Verification items for the finished model (mm, model axes). Face numbers are marked on the shaded views. A direction names the side the tool comes from. Round coordinates to 2 decimals unless told otherwise and drop trailing zeros. Write each loop counter-clockwise with the first axis right and the second up, starting at its lowest first coordinate (ties: lowest second). Pieces come first, ordered by that corner, then holes. Notation, with made-up numbers: (64.25, 75) - (113.25, 75) arc R6 ccw to (113.25, 79) - close; hole circle Ø7 at (38, 85). An arc over 180 degrees is marked (long way). Write each question's results on one line, items separated by ' | '.
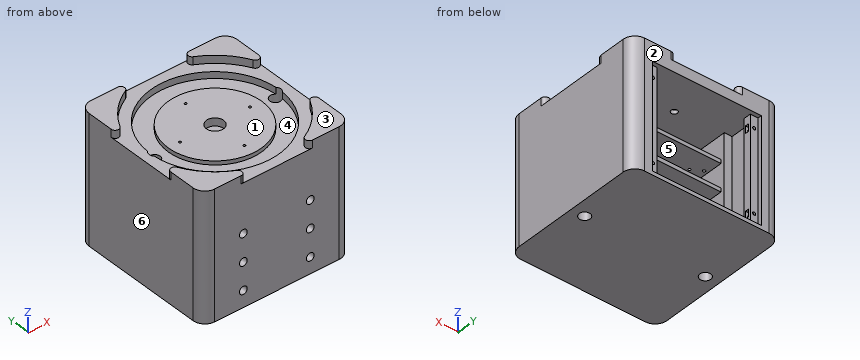
```python
from build123d import *

# Parameters (mm, degrees)
SKETCH_W             = 190
SKETCH_H             = 190
PAD_DEPTH            = 165
SKETCH001_R          = 82.5
POCKET_DEPTH         = 20
SKETCH002_R          = 60
PAD001_DEPTH         = 5
FILLET_R             = 15
SKETCH003_W          = 100
SKETCH003_H          = 30
POCKET001_DEPTH      = 160
SKETCH004_W          = 120
SKETCH004_H          = 135
POCKET002_DEPTH      = 50
SKETCH005_R          = 1.5
POCKET003_DEPTH      = 10
SKETCH006_R          = 4
POCKET004_DEPTH      = 5
SKETCH007_R          = 11
POCKET005_DEPTH      = 10
SKETCH008_W          = 140
SKETCH008_H          = 135
POCKET006_DEPTH      = 5
SKETCH009_W          = 30
SKETCH009_H          = 135
POCKET007_DEPTH      = 10
SKETCH010_W          = 30
SKETCH010_H          = 135
POCKET008_DEPTH      = 10
SKETCH011_W          = 304.305817
SKETCH011_H          = 239.475426
POCKET009_DEPTH      = 1.5
SKETCH012_R          = 96
SKETCH012_R_2        = 75
POCKET010_DEPTH      = 10
FILLET001_R          = 5
SKETCH013_R          = 2
POCKET011_DEPTH      = 10
SKETCH014_W          = 5.1
SKETCH014_H          = 9.5
POCKET012_DEPTH      = 10
SKETCH015_R          = 2
POCKET013_DEPTH      = 30.001
SKETCH016_R          = 5
POCKET014_DEPTH      = 20
SKETCH017_W          = 120
SKETCH017_H          = 30
POCKET015_DEPTH      = 110
SKETCH018_R          = 1.5
POCKET016_DEPTH      = 20
POCKET016_DEPTH_BACK = -90
SKETCH019_R          = 2
POCKET017_DEPTH      = 153.501
SKETCH020_R          = 7
POCKET018_DEPTH      = 75
SKETCH021_R          = 7
POCKET019_DEPTH      = 65
SKETCH022_W          = 10
SKETCH022_H          = 30
POCKET020_DEPTH      = 110
SKETCH023_W          = 5.1
SKETCH023_H          = 9.5
POCKET021_DEPTH      = 10
SKETCH024_R          = 1.75
POCKET022_DEPTH      = 92


with BuildPart() as part:
    # Sketch → Pad (new body)
    with BuildSketch(Plane.XY):
        Rectangle(SKETCH_W, SKETCH_H)
    extrude(amount=PAD_DEPTH)

    # Sketch001 (on Face6 of Pad) → Pocket (cut)
    with BuildSketch(Plane.XY.offset(165)):
        Circle(SKETCH001_R)
    extrude(amount=-POCKET_DEPTH, mode=Mode.SUBTRACT)

    # Sketch002 (on Face8 of Pocket) → Pad001 (join)
    with BuildSketch(Plane.XY.offset(145)):
        Circle(SKETCH002_R)
    extrude(amount=PAD001_DEPTH)

    # Fillet
    fillet_edges = [part.edges().sort_by_distance(p)[0] for p in [
        (95, -95, 82.5),
        (-95, -95, 82.5),
        (95, 95, 82.5),
        (-95, 95, 82.5),
    ]]
    fillet(fillet_edges, radius=FILLET_R)

    # Sketch003 (on Face6 of Fillet) → Pocket001 (cut)
    with BuildSketch(Plane(origin=(0, 95, 0), x_dir=(-1, 0, 0), z_dir=(0, 1, 0))):
        with Locations((0, 20)):
            Rectangle(SKETCH003_W, SKETCH003_H)
        with Locations((0, 55)):
            Rectangle(SKETCH003_W, SKETCH003_H)
        with Locations((0, 90)):
            Rectangle(SKETCH003_W, SKETCH003_H)
        with Locations((0, 125)):
            Rectangle(SKETCH003_W, SKETCH003_H)
    extrude(amount=-POCKET001_DEPTH, mode=Mode.SUBTRACT)

    # Sketch004 (on Face6 of Pocket001) → Pocket002 (cut)
    with BuildSketch(Plane(origin=(0, 95, 0), x_dir=(-1, 0, 0), z_dir=(0, 1, 0))):
        with Locations((0, 72.5)):
            Rectangle(SKETCH004_W, SKETCH004_H)
    extrude(amount=-POCKET002_DEPTH, mode=Mode.SUBTRACT)

    # Sketch005 (on Face41 of Pocket002) → Pocket003 (cut)
    with BuildSketch(Plane.XY.offset(150)):
        with Locations((0, 45)):
            Circle(SKETCH005_R)
        with Locations((45, 0)):
            Circle(SKETCH005_R)
        with Locations((0, -45)):
            Circle(SKETCH005_R)
        with Locations((-45, 0)):
            Circle(SKETCH005_R)
    extrude(amount=-POCKET003_DEPTH, mode=Mode.SUBTRACT)

    # Sketch006 (on Face21 of Pocket003) → Pocket004 (cut)
    with BuildSketch(Plane(origin=(0, 0, 140), x_dir=(1, 0, 0), z_dir=(0, 0, -1))):
        with Locations((-45, 0)):
            Circle(SKETCH006_R)
        with Locations((0, -45)):
            Circle(SKETCH006_R)
        with Locations((45, 0)):
            Circle(SKETCH006_R)
        with Locations((0, 45)):
            Circle(SKETCH006_R)
    extrude(amount=-POCKET004_DEPTH, mode=Mode.SUBTRACT)

    # Sketch007 (on Face46 of Pocket004) → Pocket005 (cut)
    with BuildSketch(Plane.XY.offset(150)):
        Circle(SKETCH007_R)
    extrude(amount=-POCKET005_DEPTH, mode=Mode.SUBTRACT)

    # Sketch008 (on Face6 of Pocket005) → Pocket006 (cut)
    with BuildSketch(Plane(origin=(0, 95, 0), x_dir=(-1, 0, 0), z_dir=(0, 1, 0))):
        with Locations((0, 72.5)):
            Rectangle(SKETCH008_W, SKETCH008_H)
    extrude(amount=-POCKET006_DEPTH, mode=Mode.SUBTRACT)

    # Sketch009 (on Face39 of Pocket006) → Pocket007 (cut)
    with BuildSketch(Plane(origin=(60, 0, 0), x_dir=(0, -1, 0), z_dir=(-1, 0, 0))):
        with Locations((-65, 72.5)):
            Rectangle(SKETCH009_W, SKETCH009_H)
    extrude(amount=-POCKET007_DEPTH, mode=Mode.SUBTRACT)

    # Sketch010 (on Face36 of Pocket007) → Pocket008 (cut)
    with BuildSketch(Plane.YZ.offset(-60)):
        with Locations((65, 72.5)):
            Rectangle(SKETCH010_W, SKETCH010_H)
    extrude(amount=-POCKET008_DEPTH, mode=Mode.SUBTRACT)

    # Sketch011 (on Face5 of Pocket008) → Pocket009 (cut)
    with BuildSketch(Plane.XY.offset(165)):
        with Locations((9.721146, 11.953617)):
            Rectangle(SKETCH011_W, SKETCH011_H)
    extrude(amount=-POCKET009_DEPTH, mode=Mode.SUBTRACT)

    # Sketch012 (on Face4 of Pocket009) → Pocket010 (cut)
    with BuildSketch(Plane.XY.offset(163.5)):
        Circle(SKETCH012_R)
        Circle(SKETCH012_R_2, mode=Mode.SUBTRACT)
    extrude(amount=-POCKET010_DEPTH, mode=Mode.SUBTRACT)

    # Fillet001
    fillet001_edges = [part.edges().sort_by_distance(p)[0] for p in [
        (-95, -13.820275, 158.5),
        (-95, 13.820275, 158.5),
        (13.820275, -95, 158.5),
        (-13.820275, -95, 158.5),
        (95, -13.820275, 158.5),
        (95, 13.820275, 158.5),
        (-13.820275, 95, 158.5),
        (13.820275, 95, 158.5),
    ]]
    fillet(fillet001_edges, radius=FILLET001_R)

    # Sketch013 (on Face44 of Fillet001) → Pocket011 (cut)
    with BuildSketch(Plane(origin=(0, 90, 0), x_dir=(-1, 0, 0), z_dir=(0, 1, 0))):
        with Locations((65, 125)):
            Circle(SKETCH013_R)
        with Locations((65, 20)):
            Circle(SKETCH013_R)
        with Locations((-65, 20)):
            Circle(SKETCH013_R)
        with Locations((-65, 125)):
            Circle(SKETCH013_R)
    extrude(amount=-POCKET011_DEPTH, mode=Mode.SUBTRACT)

    # Sketch014 (on Face53 of Pocket011) → Pocket012 (cut)
    with BuildSketch(Plane(origin=(60, 0, 0), x_dir=(0, -1, 0), z_dir=(-1, 0, 0))):
        with Locations((-85, 125)):
            Rectangle(SKETCH014_W, SKETCH014_H)
        with Locations((-85, 20)):
            Rectangle(SKETCH014_W, SKETCH014_H)
    extrude(amount=-POCKET012_DEPTH, mode=Mode.SUBTRACT)

    # Sketch015 (on Face101 of Pocket012) → Pocket013 (cut, through all)
    with BuildSketch(Plane(origin=(0, -65, 0), x_dir=(-1, 0, 0), z_dir=(0, 1, 0))):
        with Locations((-43, 91)):
            Circle(SKETCH015_R)
        with Locations((43, 91)):
            Circle(SKETCH015_R)
        with Locations((-43, 56)):
            Circle(SKETCH015_R)
        with Locations((43, 56)):
            Circle(SKETCH015_R)
        with Locations((-43, 21)):
            Circle(SKETCH015_R)
        with Locations((43, 21)):
            Circle(SKETCH015_R)
    extrude(amount=-POCKET013_DEPTH, mode=Mode.SUBTRACT)

    # Sketch016 (on Face12 of Pocket013) → Pocket014 (cut)
    with BuildSketch(Plane.XZ.offset(95)):
        with Locations((-43, 91)):
            Circle(SKETCH016_R)
        with Locations((-43, 56)):
            Circle(SKETCH016_R)
        with Locations((-43, 21)):
            Circle(SKETCH016_R)
        with Locations((43, 21)):
            Circle(SKETCH016_R)
        with Locations((43, 56)):
            Circle(SKETCH016_R)
        with Locations((43, 91)):
            Circle(SKETCH016_R)
    extrude(amount=-POCKET014_DEPTH, mode=Mode.SUBTRACT)

    # Sketch017 (on Face70 of Pocket014) → Pocket015 (cut)
    with BuildSketch(Plane(origin=(0, 45, 0), x_dir=(-1, 0, 0), z_dir=(0, 1, 0))):
        with Locations((0, 125)):
            Rectangle(SKETCH017_W, SKETCH017_H)
    extrude(amount=-POCKET015_DEPTH, mode=Mode.SUBTRACT)

    # Sketch018 (on Face124 of Pocket015) → Pocket016 (cut, two sides)
    with BuildSketch(Plane(origin=(0, 0, 105), x_dir=(1, 0, 0), z_dir=(0, 0, -1))) as pocket016_sk:
        with Locations((-42.5, -17.5)):
            Circle(SKETCH018_R)
        with Locations((-42.5, 37.5)):
            Circle(SKETCH018_R)
        with Locations((42.5, -17.5)):
            Circle(SKETCH018_R)
        with Locations((42.5, 37.5)):
            Circle(SKETCH018_R)
    extrude(amount=-POCKET016_DEPTH, mode=Mode.SUBTRACT)
    extrude(pocket016_sk.sketch, amount=-POCKET016_DEPTH_BACK, mode=Mode.SUBTRACT)

    # Sketch019 (on Face5 of Pocket016) → Pocket017 (cut, through all)
    with BuildSketch(Plane.XY.offset(153.5)):
        with Locations((-77.5, 0)):
            Circle(SKETCH019_R)
        with Locations((77.5, 0)):
            Circle(SKETCH019_R)
    extrude(amount=-POCKET017_DEPTH, mode=Mode.SUBTRACT)

    # Sketch020 (on Face5 of Pocket017) → Pocket018 (cut)
    with BuildSketch(Plane.XY.offset(153.5)):
        with Locations((-77.5, 0)):
            Circle(SKETCH020_R)
        with Locations((77.5, 0)):
            Circle(SKETCH020_R)
    extrude(amount=-POCKET018_DEPTH, mode=Mode.SUBTRACT)

    # Sketch021 (on Face6 of Pocket018) → Pocket019 (cut)
    with BuildSketch(Plane(origin=(0, 0, 0), x_dir=(1, 0, 0), z_dir=(0, 0, -1))):
        with Locations((77.5, 0)):
            Circle(SKETCH021_R)
        with Locations((-77.5, 0)):
            Circle(SKETCH021_R)
    extrude(amount=-POCKET019_DEPTH, mode=Mode.SUBTRACT)

    # Sketch022 (on Face94 of Pocket019) → Pocket020 (cut)
    with BuildSketch(Plane(origin=(0, 45, 0), x_dir=(-1, 0, 0), z_dir=(0, 1, 0))):
        with Locations((-55, 90)):
            Rectangle(SKETCH022_W, SKETCH022_H)
        with Locations((-55, 55)):
            Rectangle(SKETCH022_W, SKETCH022_H)
        with Locations((-55, 20)):
            Rectangle(SKETCH022_W, SKETCH022_H)
        with Locations((55, 20)):
            Rectangle(SKETCH022_W, SKETCH022_H)
        with Locations((55, 55)):
            Rectangle(SKETCH022_W, SKETCH022_H)
        with Locations((55, 90)):
            Rectangle(SKETCH022_W, SKETCH022_H)
    extrude(amount=-POCKET020_DEPTH, mode=Mode.SUBTRACT)

    # Sketch023 (on Face85 of Pocket020) → Pocket021 (cut)
    with BuildSketch(Plane.YZ.offset(-60)):
        with Locations((85, 20)):
            Rectangle(SKETCH023_W, SKETCH023_H)
        with Locations((85, 125)):
            Rectangle(SKETCH023_W, SKETCH023_H)
    extrude(amount=-POCKET021_DEPTH, mode=Mode.SUBTRACT)

    # Sketch024 (on Face158 of Pocket021) → Pocket022 (cut)
    with BuildSketch(Plane.XY.offset(110)):
        with Locations((55, 25)):
            Circle(SKETCH024_R)
        with Locations((55, -45)):
            Circle(SKETCH024_R)
        with Locations((-55, 25)):
            Circle(SKETCH024_R)
        with Locations((-55, -45)):
            Circle(SKETCH024_R)
    extrude(amount=-POCKET022_DEPTH, mode=Mode.SUBTRACT)


solid = part.part
```
(1) Go/stop test with flat-tipped pins: pin 1 Ø5 at (x, z) = (43, 56) entering from -Y; pin 2 Ø10 at (x, z) = (-30, 63.5) entering from +Y; pin 3 Ø11 at (x, y) = (-77.5, 0) entering from -Z. Record where each tip stops, or that it passes through.
Answer:
pin 1: y = -75 | pin 2: y = -65 | pin 3: z = 65
(2) Set-up check for the marked faces 5 and 6: record each of +Z, -Z, +X, -X, +Y, -Y from which the full face is reachable in a straight line by a thin tool's end or side.
Answer:
face 5: +Y | face 6: +Z, -Z, -X, +Y, -Y
(3) Thickness scan on L1, parallel to Z at x = -50.5, y = -44.5; L2, parallel to Z at x = 16, y = 32; L3, parallel to Y at x = -42.5, z = 71.35. Record the ranges inside material, lowest first.
Answer:
L1: 0 to 5, 35 to 40, 70 to 75, 105 to 110, 140 to 145 | L2: 0 to 5, 35 to 40, 70 to 75, 105 to 110, 140 to 150 | L3: -95 to -39, -36 to 16, 19 to 45
(4) Section check A-A (z = 133). Record the cut outline in (x, y).
Answer:
outline: (-95, -80) arc R15 ccw to (-80, -95) - (80, -95) arc R15 ccw to (95, -80) - (95, 80) arc R15 ccw to (80, 95) - (70, 95) - (70, 90) - (60, 90) - (60, 80) - (70, 80) - (70, 50) - (60, 50) - (60, -65) - (-60, -65) - (-60, 50) - (-70, 50) - (-70, 80) - (-60, 80) - (-60, 90) - (-70, 90) - (-70, 95) - (-80, 95) arc R15 ccw to (-95, 80) - close; hole circle Ø14 at (-77.5, 0); hole circle Ø14 at (77.5, 0)
(5) Section check B-B (x = 31). Record the cut outline in (y, z), plus the area to 3 significant figures.
Answer:
outline: (-95, 0) - (95, 0) - (95, 5) - (-65, 5) - (-65, 35) - (45, 35) - (45, 40) - (-65, 40) - (-65, 70) - (45, 70) - (45, 75) - (-65, 75) - (-65, 105) - (45, 105) - (45, 110) - (-65, 110) - (-65, 140) - (95, 140) - (95, 153.5) - (76.45, 153.5) - (76.45, 145) - (51.37, 145) - (51.37, 150) - (-51.37, 150) - (-51.37, 145) - (-76.45, 145) - (-76.45, 153.5) - (-95, 153.5) - close | area: 8,430 mm2
(6) Mould release check, pull along Y, two halves, no side actions. Record for the marked faces 1, 2, 3 and 4: released by +Y, released by -Y, zero draft, split by the parting line, or undercut.
Answer:
face 1: undercut | face 2: released by +Y | face 3: zero draft | face 4: undercut
